Model file for the job. Use its own axes, mm. A direction names the side the tool comes from. Round coordinates to 2 decimals unless told otherwise and drop trailing zeros. Loops run counter-clockwise (first coordinate to the right, second up) from the corner with the lowest first, then second, coordinate; pieces in that order, holes last.
from build123d import *

# Parameters (mm, degrees)
SKETCH1_R                        = 3.35
BOSS_EXTRUDE1_DEPTH              = 12
BOSS_EXTRUDE4_DEPTH              = 23
CUT_EXTRUDE2_DEPTH               = 227.564419348
BOSS_EXTRUDE5_DEPTH              = 22
RIB8_REACH                       = 234.673
SKETCH9_WALL_W                   = 590.286406192
SKETCH9_WALL_H                   = 8
RIB13_REACH                      = 234.673
SKETCH10_WALL_W                  = 582.229830078
SKETCH10_WALL_H                  = 6
F_25_64_0_39063_DIAMETER_HOLE1_D = 9.922002


with BuildPart() as part:
    # Sketch1 → Boss-Extrude1 (new body)
    with BuildSketch(Plane.XY):
        Polygon((0, 0), (-40.842464086, 0), (-68.59, 50), (-68.59, 85), (0, 85), align=None)
        with Locations((-30.59, 42)):
            Circle(SKETCH1_R, mode=Mode.SUBTRACT)
        with Locations((-16.59, 42)):
            Circle(SKETCH1_R, mode=Mode.SUBTRACT)
        with Locations((-24, 10)):
            Circle(SKETCH1_R, mode=Mode.SUBTRACT)
        with Locations((-10, 10)):
            Circle(SKETCH1_R, mode=Mode.SUBTRACT)
        with BuildLine():
            Line((-45.24, 60), (-45.24, 54))
            ThreePointArc((-45.24, 54), (-48.59, 50.65), (-51.94, 54))
            Line((-51.94, 54), (-51.94, 60))
            ThreePointArc((-51.94, 60), (-48.59, 63.35), (-45.24, 60))
        make_face(mode=Mode.SUBTRACT)
        with BuildLine():
            Line((-45.24, 78), (-45.24, 72))
            ThreePointArc((-45.24, 72), (-48.59, 68.65), (-51.94, 72))
            Line((-51.94, 72), (-51.94, 78))
            ThreePointArc((-51.94, 78), (-48.59, 81.35), (-45.24, 78))
        make_face(mode=Mode.SUBTRACT)
        with BuildLine():
            Line((-27.24, 78), (-27.24, 72))
            ThreePointArc((-27.24, 72), (-30.59, 68.65), (-33.94, 72))
            Line((-33.94, 72), (-33.94, 78))
            ThreePointArc((-33.94, 78), (-30.59, 81.35), (-27.24, 78))
        make_face(mode=Mode.SUBTRACT)
        with BuildLine():
            Line((-27.24, 60), (-27.24, 54))
            ThreePointArc((-27.24, 54), (-30.59, 50.65), (-33.94, 54))
            Line((-33.94, 54), (-33.94, 60))
            ThreePointArc((-33.94, 60), (-30.59, 63.35), (-27.24, 60))
        make_face(mode=Mode.SUBTRACT)
    extrude(amount=BOSS_EXTRUDE1_DEPTH)

    # Sketch4 → Boss-Extrude4 (add)
    with BuildSketch(Plane.ZY.offset(68.59)):
        with BuildLine():
            Line((1.350364369, 200.289400401), (-0.475324009, 200.094696819))
            Line((-0.475324009, 200.094696819), (-0.475324009, 198.169964836))
            Line((-0.475324009, 198.169964836), (-0.475324009, 196.253602357))
            add(Edge.make_bspline(
                [(-0.475324009, 196.253602357), (-0.475324009, 196.12869199), (-0.518289538, 195.884432771), (-0.746214851, 195.524493199), (-1.106154424, 195.296567886), (-1.350413642, 195.253602357), (-1.475324009, 195.253602357)],
                knots=[0, 0, 0, 0, 0.25, 0.5, 0.75, 1, 1, 1, 1], degree=3))
            Line((-1.475324009, 195.253602357), (-45.975324009, 195.253602357))
            Line((-45.975324009, 195.253602357), (-45.975324009, 208.004109944))
            Line((-45.975324009, 208.004109944), (23.394468779, 208.004109944))
            Line((23.394468779, 208.004109944), (12, 85))
            Line((12, 85), (2.281711333, 85))
            Line((2.281711333, 85), (5.872362287, 123.761337788))
            Line((5.872362287, 123.761337788), (12.546460431, 195.808707235))
            Line((12.546460431, 195.808707235), (12.52462737, 198.022692939))
            add(Edge.make_bspline(
                [(12.52462737, 198.022692939), (12.52275101, 198.212965603), (12.485055554, 198.584771055), (12.246945435, 199.373301804), (11.607215228, 200.288314456), (10.634477398, 200.836296213), (9.82657242, 200.996816362), (9.452863838, 200.998278344), (9.263306003, 200.981694182)],
                knots=[0, 0, 0, 0, 0.125, 0.25, 0.5, 0.75, 0.875, 1, 1, 1, 1], degree=3))
            Line((9.263306003, 200.981694182), (1.350364369, 200.289400401))
        make_face()
    extrude(amount=-BOSS_EXTRUDE4_DEPTH)

    # Sketch6 → Cut-Extrude2 (cut, through all)
    with BuildSketch(Plane.XY.offset(12)):
        Polygon((-16.781583806, 99.760607563), (-7.709196228, 49.999997515), (7.428297799, 49.999995871), (-1.644090079, 99.760607563), align=None)
    extrude(amount=-CUT_EXTRUDE2_DEPTH, mode=Mode.SUBTRACT)

    # Sketch7 → Boss-Extrude5 (add)
    with BuildSketch(Plane.ZY.offset(68.59)):
        with BuildLine():
            Line((1.350364369, 200.289400401), (9.263306003, 200.981694182))
            add(Edge.make_bspline(
                [(9.263306003, 200.981694182), (9.452863838, 200.998278344), (9.82657242, 200.996816362), (10.634477398, 200.836296213), (11.607215228, 200.288314456), (12.246945435, 199.373301804), (12.485055554, 198.584771055), (12.52275101, 198.212965603), (12.52462737, 198.022692939)],
                knots=[0, 0, 0, 0, 0.125, 0.25, 0.5, 0.75, 0.875, 1, 1, 1, 1], degree=3))
            Line((12.52462737, 198.022692939), (12.546460431, 195.808707235))
            Line((12.546460431, 195.808707235), (11.914066265, 188.98196658))
            Line((11.914066265, 188.98196658), (21.549669936, 188.089373761))
            Line((21.549669936, 188.089373761), (23.394468779, 208.004109944))
            Line((23.394468779, 208.004109944), (-45.975324009, 208.004109944))
            Line((-45.975324009, 208.004109944), (-45.975324009, 195.253602357))
            Line((-45.975324009, 195.253602357), (-1.475324009, 195.253602357))
            add(Edge.make_bspline(
                [(-1.475324009, 195.253602357), (-1.350413642, 195.253602357), (-1.106154424, 195.296567886), (-0.746214851, 195.524493199), (-0.518289538, 195.884432771), (-0.475324009, 196.12869199), (-0.475324009, 196.253602357)],
                knots=[0, 0, 0, 0, 0.25, 0.5, 0.75, 1, 1, 1, 1], degree=3))
            Line((-0.475324009, 196.253602357), (-0.475324009, 200.094696819))
            Line((-0.475324009, 200.094696819), (1.350364369, 200.289400401))
        make_face()
    extrude(amount=BOSS_EXTRUDE5_DEPTH)

    # Sketch9 wall → Rib8 (add, up to next)
    with BuildSketch(Plane(origin=(-79.59, 127.869133691, 15.971176294), x_dir=(0.178948228267, -0.979664115124, -0.090751050339), z_dir=(0.983858491654, 0.178185337816, 0.016506174221)), mode=Mode.PRIVATE) as rib8_sk1:
        with Locations((0, 4)):
            Rectangle(SKETCH9_WALL_W, SKETCH9_WALL_H)
    rib8_tool1 = extrude(rib8_sk1.sketch, amount=RIB8_REACH, mode=Mode.PRIVATE) - part.part
    add(rib8_tool1.solids().sort_by_distance((-79.59, 127.869133691, 15.971176294))[0])

    # Sketch10 wall → Rib13 (add, up to next)
    with BuildSketch(Plane(origin=(-34.166372331, 141.054628888, 17.192612824), x_dir=(0.198872370592, -0.975847362421, -0.090397485977), z_dir=(0.98002539774, 0.198024539719, 0.018343975956)), mode=Mode.PRIVATE) as rib13_sk1:
        with Locations((0, 3)):
            Rectangle(SKETCH10_WALL_W, SKETCH10_WALL_H)
    rib13_tool1 = extrude(rib13_sk1.sketch, amount=-RIB13_REACH, mode=Mode.PRIVATE) - part.part
    add(rib13_tool1.solids().sort_by_distance((-34.166372331, 141.054628888, 17.192612824))[0])

    # 25/64 (0.39063) Diameter Hole1 (through all)
    with Locations(Plane(origin=(0, 208.004109944, 0), x_dir=(1, 0, 0), z_dir=(0, 1, 0))):
        with Locations((-68.242097157, 23.725324009)):
            Hole(F_25_64_0_39063_DIAMETER_HOLE1_D / 2)


solid = part.part
Q1. Probe line 1 (Y direction, x = -17, z = 5.5); line 2 (Y direction, x = -28, z = 5.5); line 3 (Z direction, x = -53.5, y = 40). List the from-to ranges inside material, lowest first.
Q2. Slice it at C-C on y = 10. Give the cut face in (x, z).
Q3. Flat gauge pins, fed straight in: P1, Ø11, axis at y = 109.5, z = 8, coming from the -X side; P2, Ø3, axis at y = 76, z = 5.5, coming from the +X side; P3, Ø3, axis at y = 57.5, z = 7, coming from the +X side. Where does each tip first touch, or does it go through?
Q4. Slice it at D-D on y = 102.5. Give the cut face in (x, z).
Q5. Tool access for faces 1 (the face through (-40.14, 127.9, 9.95)), 2 (the face through (-67.78, 200.63, 5.25)), 3 (the face through (-48.52, 68.65, 5.92)): list every direction of +Z, -Z, +X, -X, +Y, -Y with a clear straight run to the whole face (end or side of a thin tool).
Q6. Slice it at B-B on x = -30.59. Give the cut face in (y, z).
Q7. Slice it at A-A on x = -10. Give the cut face in (y, z).
Q8. Pull direction Z, two halves, no side cores. Call faces 4 (the face through (-30.52, 50.65, 5.92)), 5 (the face through (-72.825, 201.54, -21.825)), 6 (the face through (-74.06, 144.31, 9.46)): pulls with the +Z half, pulls with the -Z half, needs draft (parallel to the pull), parting line crosses it, or undercut.
Reply:
1. line 1: y = 0 to 38.68, 45.32 to 85
1. line 2: y = 0 to 39.88, 44.12 to 51.88, 62.12 to 69.88, 80.12 to 85
1. line 3: z = 0 to 12
2. outline: (-46.39, 0) - (-27.35, 0) - (-27.35, 12) - (-46.39, 12) - close; (-20.65, 0) - (-13.35, 0) - (-13.35, 12) - (-20.65, 12) - close; (-6.65, 0) - (0, 0) - (0, 12) - (-6.65, 12) - close
3. P1: stops at x = -77.13
3. P2: stops at x = -12.18
3. P3: stops at x = -8.8
4. outline: (-74.96, 13.62) - (-74.82, 5.59) - (-68.59, 5.59) - (-68.59, 3.9) - (-45.59, 3.9) - (-45.59, 7.6) - (-26.2, 7.6) - (-26.31, 13.62) - close
5. face 1: -Z, +X, +Y
5. face 2: +X, -X
5. face 3: +Z, -Z
6. outline: (0, 0) - (38.65, 0) - (38.65, 12) - (0, 12) - close; (45.35, 0) - (50.65, 0) - (50.65, 12) - (45.35, 12) - close; (63.35, 0) - (68.65, 0) - (68.65, 12) - (63.35, 12) - close; (81.35, 0) - (85, 0) - (85, 5.97) - (124.06, 9.59) - (123.51, 15.57) - (85, 12) - (81.35, 12) - close
7. outline: (0, 0) - (6.65, 0) - (6.65, 12) - (0, 12) - close; (13.35, 0) - (62.56, 0) - (62.56, 12) - (13.35, 12) - close
8. face 4: needs draft
8. face 5: undercut
8. face 6: pulls with the -Z half
